Could you check a few things on this model? Use its own coordinates, in mm. A direction names the side the tool comes from. Coordinates: 2 decimals unless noted, no trailing zeros. Write each loop counter-clockwise with the first axis right and the second up, starting at its lowest first coordinate (ties: lowest second). Pieces come first, ordered by that corner, then holes. Notation, with made-up numbers: (-6, 5) - (44, 5) arc R15 ccw to (44, 26) - close; hole circle Ø8 at (33, 23). An arc over 180 degrees is marked (long way). Answer as a JSON object with one key per item and string values. Group by question number.
1) Please list where these lines run through material, in increasing order: line 1 along Z through (x, y) = (-83, -2.1); line 2 along X through (y, z) = (-1.05, -17); line 3 along Z through (x, y) = (-4.5, -0.25).
2) If we section it at C-C (z = -43): Write out the boundary of the cut face in (x, y), plus the area to 3 significant figures.
3) If we section it at A-A (z = -62): Write out the boundary of the cut face in (x, y).
4) If we section it at D-D (y = -1.1): Write out the boundary of the cut face in (x, z), plus the area to 3 significant figures.
5) On a 3-axis mill with a long thin cutter (end or side, diameter ignored), from which of +Z, -Z, +X, -X, +Y, -Y can I reach the whole of each face in a straight line? I mean faces 4 (the cylindrical face through (-77.15, -2.96, 56.99)), 5 (the flat face through (-1, -3, -70)). Say none if no direction works.
6) We'd pull the mould along X, two halves only. Please class faces 1 (the flat face through (90, -3, -1)), 2 (the flat face through (-7, 0, 63)), 3 (the cylindrical face through (-81.925, -3.042, 63.686)): released by +X, released by -X, zero draft, split by the parting line, or undercut.
7) If we section it at B-B (x = 47.5): Write out the boundary of the cut face in (y, z).
```python
from build123d import *

# Parameters (mm, degrees)
F1_DEPTH = 6
F2_R     = 2
F3_DEPTH = 25


with BuildPart() as f1:
    # F0 (on Front) → F1 (new body)
    with BuildSketch(Plane.XZ):
        with BuildLine():
            Line((-90, 70), (-90, -70))
            Line((-90, -70), (90, -70))
            Line((90, -70), (90, 0))
            Line((90, 0), (80, 0))
            Line((80, 0), (80, -50))
            ThreePointArc((80, -50), (77.071068, -57.071068), (70, -60))
            Line((70, -60), (-70, -60))
            ThreePointArc((-70, -60), (-77.071068, -57.071068), (-80, -50))
            Line((-80, -50), (-80, 50))
            ThreePointArc((-80, 50), (-77.071068, 57.071068), (-70, 60))
            Line((-70, 60), (0, 60))
            Line((0, 60), (0, 70))
            Line((0, 70), (-90, 70))
        make_face()
        with BuildLine():
            Line((80, 0), (90, 0))
            Line((90, 0), (90, 70))
            Line((90, 70), (0, 70))
            Line((0, 70), (0, 60))
            Line((0, 60), (70, 60))
            ThreePointArc((70, 60), (77.071068, 57.071068), (80, 50))
            Line((80, 50), (80, 0))
        make_face()
    extrude(amount=F1_DEPTH)

    # F2 (on face) → F3 (cut)
    with BuildSketch(Plane.XZ.offset(6)):
        with Locations((-83, 62)):
            Circle(F2_R)
        with Locations((-83, -62)):
            Circle(F2_R)
        with Locations((83, -62)):
            Circle(F2_R)
        with Locations((83, 62)):
            Circle(F2_R)
    extrude(amount=-F3_DEPTH, mode=Mode.SUBTRACT)


solid = f1.part
```
Here are the results:
{
 "1": {"line 1": "z = -70 to -64, -60 to 60, 64 to 70", "line 2": "x = -90 to -80, 80 to 90", "line 3": "z = -70 to -60, 60 to 70"},
 "2": {"outline": "(-90, -6) - (-80, -6) - (-80, 0) - (-90, 0) - close; (80, -6) - (90, -6) - (90, 0) - (80, 0) - close", "area": "120 mm²"},
 "3": {"outline": "(-90, -6) - (-85, -6) - (-85, 0) - (-90, 0) - close; (-81, -6) - (81, -6) - (81, 0) - (-81, 0) - close; (85, -6) - (90, -6) - (90, 0) - (85, 0) - close"},
 "4": {"outline": "(-90, -70) - (90, -70) - (90, 70) - (-90, 70) - close; hole circle Ø4 at (-83, -62); hole circle Ø4 at (-83, 62); hole (-80, -50) arc R10 ccw to (-70, -60) - (70, -60) arc R10 ccw to (80, -50) - (80, 50) arc R10 ccw to (70, 60) - (-70, 60) arc R10 ccw to (-80, 50) - close; hole circle Ø4 at (83, -62); hole circle Ø4 at (83, 62)", "area": "6,040 mm²"},
 "5": {"face 4": "+Y, -Y", "face 5": "-Z, +X, -X, +Y, -Y"},
 "6": {"face 1": "released by +X", "face 2": "zero draft", "face 3": "undercut"},
 "7": {"outline": "(-6, -70) - (0, -70) - (0, -60) - (-6, -60) - close; (-6, 60) - (0, 60) - (0, 70) - (-6, 70) - close"}
}
